Check sheet for the modelled part. Datum: model origin and axes. Units: mm. Face numbers are marked on the shaded views. A direction names the side the tool comes from. Coordinates: 2 decimals unless noted, no trailing zeros. Loops run counter-clockwise (first coordinate to the right, second up) from the corner with the lowest first, then second, coordinate; pieces in that order, holes last. Notation, with made-up numbers: M -36.5,87.25 L -8.5,87.25 A19 cw -8.5,95.25 Z; hole C 36.25,36.5 d9. An arc over 180 degrees is marked long. Return JSON: item names as keys, results as strings.
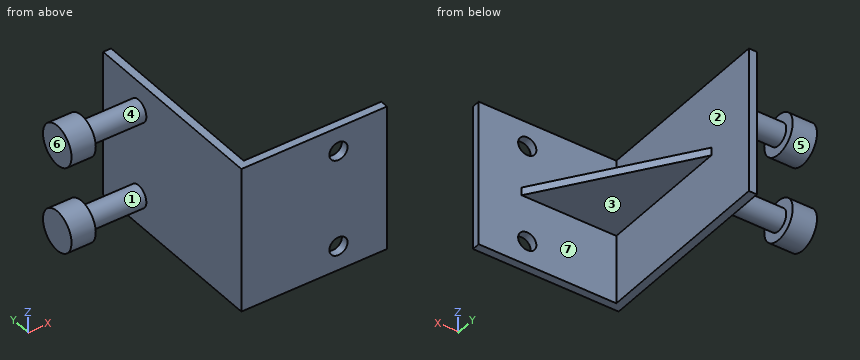
from build123d import *

# Parameters (mm, degrees)
BOSS_EXTRUDE1_DEPTH = 15.24
BOSS_EXTRUDE2_DEPTH = 0.8255
SKETCH3_R           = 1.905
CUT_EXTRUDE1_DEPTH  = 2.6764
SKETCH5_R           = 2.286
BOSS_EXTRUDE3_DEPTH = 11.938
SKETCH6_R           = 4.191
BOSS_EXTRUDE4_DEPTH = 5.08


with BuildPart() as part:
    # Sketch1 → Boss-Extrude1 (new body, symmetric)
    with BuildSketch(Plane.XY):
        Polygon((0, 0), (30.48, 0), (30.48, 1.6764), (1.6764, 1.6764), (1.6764, 40.64), (0, 40.64), align=None)
    extrude(amount=BOSS_EXTRUDE1_DEPTH, both=True)

    # Sketch2 → Boss-Extrude2 (add, symmetric)
    with BuildSketch(Plane.XY):
        Polygon((1.6764, 29.6164), (21.4884, 1.6764), (1.6764, 1.6764), align=None)
    extrude(amount=BOSS_EXTRUDE2_DEPTH, both=True)

    # Sketch3 → Cut-Extrude1 (cut, through all)
    with BuildSketch(Plane(origin=(0, 1.6764, 0), x_dir=(1, 0, 0), z_dir=(0, 1, 0))):
        with Locations((20.32, 10.16)):
            Circle(SKETCH3_R)
        with Locations((20.32, -10.16)):
            Circle(SKETCH3_R)
    extrude(amount=-CUT_EXTRUDE1_DEPTH, mode=Mode.SUBTRACT)

    # Sketch5 → Boss-Extrude3 (add)
    with BuildSketch(Plane.ZY):
        with Locations((-9.144, 30.226)):
            Circle(SKETCH5_R)
        with Locations((9.144, 30.226)):
            Circle(SKETCH5_R)
    extrude(amount=BOSS_EXTRUDE3_DEPTH)

    # Sketch6 → Boss-Extrude4 (add)
    with BuildSketch(Plane.ZY.offset(11.938)):
        with Locations((-9.144, 30.226)):
            Circle(SKETCH6_R)
        with Locations((9.144, 30.226)):
            Circle(SKETCH6_R)
    extrude(amount=BOSS_EXTRUDE4_DEPTH)


solid = part.part
1) Scan lines: line 1 along Z through (x, y) = (20.32, 1.3) (3 decimals); line 2 along X through (y, z) = (0.9, -10.16) (3 decimals); line 3 along Y through (x, z) = (17.5, 7.5). Record each from-to range of solid material in increasing order. Write a range as [from, to].
Answers:
{"line 1": "[-15.24, -12.065], [-8.255, 8.255], [12.065, 15.24]", "line 2": "[0, 18.415], [22.225, 30.48]", "line 3": "[0, 1.68]"}
2) Section check D-D on z = 3. Record the cut outline in (x, y), then the cut area to 3 significant figures.
Answers:
{"outline": "M 0,0 L 30.48,0 L 30.48,1.68 L 1.68,1.68 L 1.68,40.64 L 0,40.64 Z", "area": "116 mm²"}
3) Set-up check for the marked faces 5, 6 and 7: record each of +Z, -Z, +X, -X, +Y, -Y from which the full face is reachable in a straight line by a thin tool's end or side.
Answers:
{"face 5": "-X", "face 6": "+Z, -Z, -X, +Y, -Y", "face 7": "+X, +Y"}
4) Section check C-C on y = 25. Record the cut outline in (x, z), then the cut area to 3 significant figures.
Answers:
{"outline": "M 0,-15.24 L 1.68,-15.24 L 1.68,-0.83 L 4.95,-0.83 L 4.95,0.83 L 1.68,0.83 L 1.68,15.24 L 0,15.24 Z", "area": "56.5 mm²"}
5) Section check B-B on z = -9. Record the cut outline in (x, y).
Answers:
{"outline": "M -17.02,26.04 L -11.94,26.04 L -11.94,27.94 L 0,27.94 L 0,0 L 18.81,0 L 18.81,1.68 L 1.68,1.68 L 1.68,40.64 L 0,40.64 L 0,32.51 L -11.94,32.51 L -11.94,34.41 L -17.02,34.41 Z; M 21.83,0 L 30.48,0 L 30.48,1.68 L 21.83,1.68 Z"}
6) Go/stop test with flat-tipped pins: pin 1 Ø1.5 at (x, y) = (11.5, 10) entering from -Z; pin 2 Ø16 at (x, y) = (8.5, 17) entering from -Z; pin 3 Ø5 at (x, z) = (20.32, 10.16) entering from +Y; pin 4 Ø8 at (x, y) = (-10.5, 25.5) entering from -Z. Record where each tip stops, or that it passes through.
Answers:
{"pin 1": "z = -0.83", "pin 2": "z = -15.24", "pin 3": "y = 1.68", "pin 4": "z = -13.22"}
7) Section check A-A on x = 20.32. Record the cut outline in (y, z) (1 decimal), then the cut area to 3 significant figures.
Answers:
{"outline": "M 0,-15.2 L 1.7,-15.2 L 1.7,-12.1 L 0,-12.1 Z; M 0,-8.3 L 1.7,-8.3 L 1.7,-0.8 L 3.3,-0.8 L 3.3,0.8 L 1.7,0.8 L 1.7,8.3 L 0,8.3 Z; M 0,12.1 L 1.7,12.1 L 1.7,15.2 L 0,15.2 Z", "area": "41.0 mm²"}
8) Draft check along Z on the marked faces 1, 2, 3 and 4. Enter one of: +Z half, -Z half, draft (parallel to the pull), parting line (faces both ways), or undercut.
Answers:
{"face 1": "undercut", "face 2": "draft", "face 3": "-Z half", "face 4": "undercut"}
